Input: dimensioned drawing with shaded views. Units: mm. Origin: part minimum x, y, z. A direction names the side the tool comes from. Give positions to 0.01 mm unless a question says otherwise; leave off trailing zeros. Loops run counter-clockwise (first coordinate to the right, second up) from the corner with the lowest first, then second, coordinate; pieces in that order, holes last. Notation, with made-up numbers: (7, 43) -> (25, 43) arc R28 ccw to (25, 68) -> close; hole circle Ø4 at (67.25, 40). An arc over 180 degrees is marked (long way). Answer in a Markdown table with one row per item. Add a question column.
1) Section query C-C (y = 7). Return the cut outline in (x, z).
2) Section query A-A (x = 25). Return the cut outline in (y, z).
3) First-contact query: P1, Ø3.5, axis at y = 7, z = 10, coming from the -X side; P2, Ø12, axis at x = 12.5, z = 17, coming from the -Y side; P3, Ø6, axis at y = 22, z = 10, coming from the +X side. Flat tips, straight axial feed; report the tip coordinate or a pass-through.
4) Line query: line 1 (Y direction, x = 2, z = 10); line 2 (Y direction, x = 32, z = 13.5); line 3 (X direction, y = 8, z = 17.75). Output: solid intervals per line, ascending. Write a range as from..to.
5) Access query for the marked faces 1, 2 and 3. Directions: +Z, -Z, +X, -X, +Y, -Y. A direction counts if a zero-diameter tool reaches every point of the face in a straight line with its end or side. Return the directions, or none.
6) Section query B-B (y = 31). Return the cut outline in (x, z) (1 decimal).
7) Draft query along X for the marked faces 4, 5, 6 and 7. Return one class per face: +X half, -X half, draft (parallel to the pull), parting line (faces both ways), or undercut.
8) Section query D-D (z = 11). Return the cut outline in (x, y).
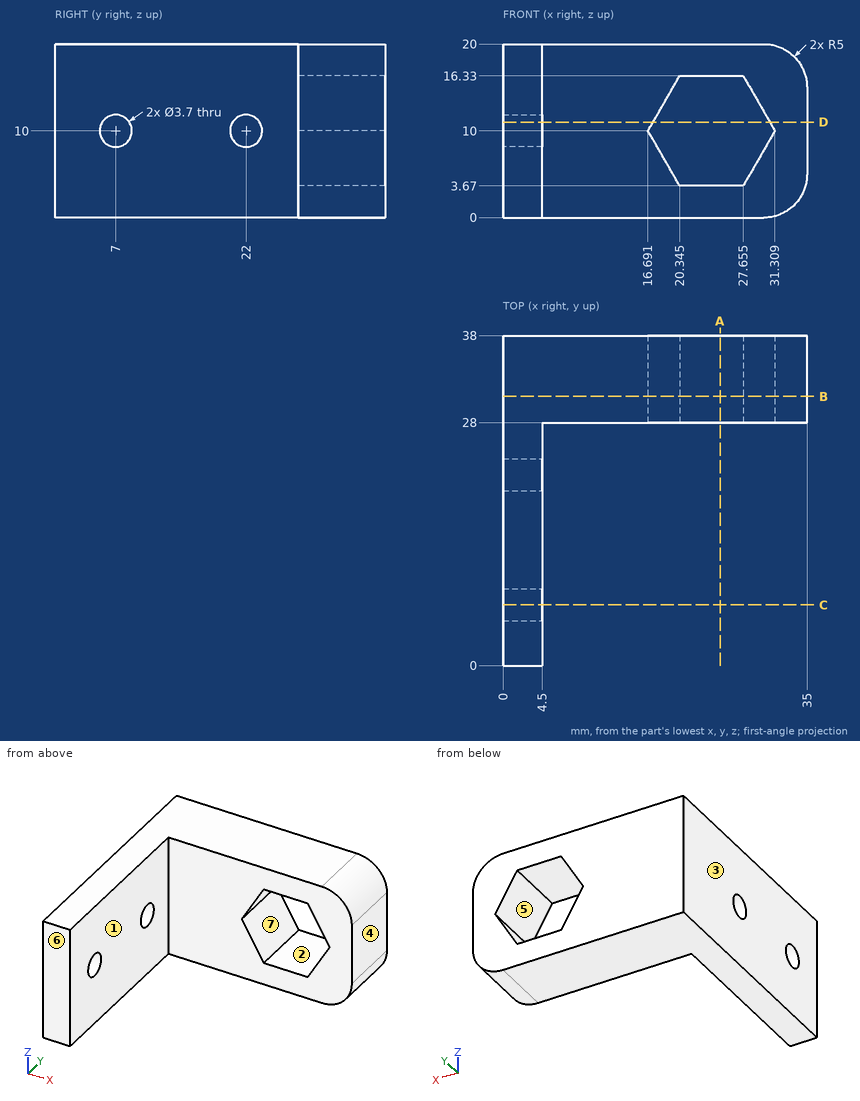
Evaluation:
| question | item | result |
|---|---|---|
| 1 | outline | (0, 0) -> (4.5, 0) -> (4.5, 8.15) -> (0, 8.15) -> close; (0, 11.85) -> (4.5, 11.85) -> (4.5, 20) -> (0, 20) -> close |
| 2 | outline | (28, 0) -> (38, 0) -> (38, 3.67) -> (28, 3.67) -> close; (28, 16.33) -> (38, 16.33) -> (38, 20) -> (28, 20) -> close |
| 3 | P1 | through |
| 3 | P2 | y = 28 |
| 3 | P3 | x = 4.5 |
| 4 | line 1 | 0..5.15, 8.85..20.15, 23.85..38 |
| 4 | line 2 | 28..38 |
| 4 | line 3 | 0..4.5 |
| 5 | face 1 | +Z, -Z, +X, -Y |
| 5 | face 2 | +Y, -Y |
| 5 | face 3 | +Z, -Z, -X, +Y, -Y |
| 6 | outline | (0, 0) -> (30, 0) arc R5 ccw to (35, 5) -> (35, 15) arc R5 ccw to (30, 20) -> (0, 20) -> close; hole (16.7, 10) -> (20.3, 3.7) -> (27.7, 3.7) -> (31.3, 10) -> (27.7, 16.3) -> (20.3, 16.3) -> close |
| 7 | face 4 | +X half |
| 7 | face 5 | undercut |
| 7 | face 6 | draft |
| 7 | face 7 | undercut |
| 8 | outline | (0, 0) -> (4.5, 0) -> (4.5, 5.44) -> (0, 5.44) -> close; (0, 8.56) -> (4.5, 8.56) -> (4.5, 20.44) -> (0, 20.44) -> close; (0, 23.56) -> (4.5, 23.56) -> (4.5, 28) -> (17.27, 28) -> (17.27, 38) -> (0, 38) -> close; (30.73, 28) -> (35, 28) -> (35, 38) -> (30.73, 38) -> close |
